Part model, mm, in its own coordinate system. A direction names the side the tool comes from. Round coordinates to 2 decimals unless told otherwise and drop trailing zeros. Loops run counter-clockwise (first coordinate to the right, second up) from the corner with the lowest first, then second, coordinate; pieces in that order, holes last. Notation, with made-up numbers: M -16.5,53.5 L 1.5,53.5 A20 ccw 1.5,74.5 Z; hole C 44.25,13.25 d1. An arc over 180 degrees is marked long. Put each result on its own line as item: value. Start each with the question number.
```python
from build123d import *
from build123d.topology import SkipClean

# Parameters (mm, degrees)
SKETCH_1_W          = 60
SKETCH_1_H          = 20
SKETCH_1_R          = 2.75
SKETCH_1_R_2        = 1.75
EXTRUDE_1_DEPTH     = 4
SKETCH_2_W          = 4
SKETCH_2_H          = 20
EXTRUDE_2_DEPTH     = 24
EXTRUDE_3_DEPTH     = 4
EXTRUDE_4_DEPTH     = 4
EXTRUDE_START       = 15
SKETCH_5_W          = 45
SKETCH_5_H          = 20
SKETCH_5_R          = 1.75
EXTRUDE_5_DEPTH     = 15
SKETCH_6_W          = 40
SKETCH_6_H          = 12
CUT_EXTRUDE_1_DEPTH = 15
SKETCH_7_R          = 2.75
CUT_EXTRUDE_2_DEPTH = 15
CUT_EXTRUDE_3_REACH = 76.303
SKETCH_8_W          = 30
SKETCH_8_H          = 20
SKETCH_10_W         = 26
SKETCH_10_H         = 12
EXTRUDE_6_DEPTH     = 4
SKETCH_11_W         = 15
SKETCH_11_H         = 12
EXTRUDE_7_DEPTH     = 4


with BuildPart() as part:
    # 草图1 → 凸台-拉伸1 (new body)
    with BuildSketch(Plane.XY):
        with Locations((30, -10)):
            Rectangle(SKETCH_1_W, SKETCH_1_H)
        with Locations((5, -5)):
            Circle(SKETCH_1_R, mode=Mode.SUBTRACT)
        with Locations((5, -15)):
            Circle(SKETCH_1_R, mode=Mode.SUBTRACT)
        with Locations((55, -10)):
            Circle(SKETCH_1_R_2, mode=Mode.SUBTRACT)
    extrude(amount=EXTRUDE_1_DEPTH)

    # 草图2 → 凸台-拉伸2 (add)
    with BuildSketch(Plane(origin=(0, 0, 0), x_dir=(-1, 0, 0), z_dir=(0, 0, -1))):
        with Locations((-17, -10)):
            Rectangle(SKETCH_2_W, SKETCH_2_H)
    extrude(amount=-EXTRUDE_2_DEPTH)

    # 草图3 → 凸台-拉伸3 (add)
    with BuildSketch(Plane.XZ.offset(20)):
        Polygon((19, 24), (60, 4), (19, 4), align=None)
    extrude(amount=-EXTRUDE_3_DEPTH)

    # 草图4 → 凸台-拉伸4 (add)
    with BuildSketch(Plane(origin=(0, 0, 0), x_dir=(1, 0, 0), z_dir=(0, 1, 0))):
        Polygon((19, -24), (60, -4), (19, -4), align=None)
    extrude(amount=-EXTRUDE_4_DEPTH)

    # 草图5 → 凸台-拉伸5 (add)
    with SkipClean():  # the faces are left unmerged after this step: merging them gives an invalid solid
        with BuildSketch(Plane(origin=(0, 0, 0), x_dir=(-1, 0, 0), z_dir=(0, 0, -1)).offset(EXTRUDE_START)):
            with Locations((-37.5, -10)):
                Rectangle(SKETCH_5_W, SKETCH_5_H)
            with Locations((-55, -10)):
                Circle(SKETCH_5_R, mode=Mode.SUBTRACT)
        extrude(amount=-EXTRUDE_5_DEPTH)

    # 草图6 → 切除-拉伸1 (cut)
    with BuildSketch(Plane.XY.offset(4)):
        with Locations((40, -10)):
            Rectangle(SKETCH_6_W, SKETCH_6_H)
    extrude(amount=-CUT_EXTRUDE_1_DEPTH, mode=Mode.SUBTRACT)

    # 草图7 → 切除-拉伸2 (cut)
    with BuildSketch(Plane(origin=(19, 0, 0), x_dir=(0, 0, -1), z_dir=(1, 0, 0))):
        with Locations(Location((-14, -10, 0), (0, 0, 90))):
            Circle(SKETCH_7_R)
    extrude(amount=-CUT_EXTRUDE_2_DEPTH, mode=Mode.SUBTRACT)

    # 切除-拉伸3: up to this face of the body (flat: up to its plane)
    cut_extrude_3_end = Plane(part.part.faces().sort_by_distance((7.970492187, -10, 0))[0])
    # 草图8 → 切除-拉伸3 (cut, up to the picked face)
    with BuildSketch(Plane(origin=(0, 0, -15), x_dir=(-1, 0, 0), z_dir=(0, 0, -1)), mode=Mode.PRIVATE) as cut_extrude_3_sk1:
        with Locations((-30, -10)):
            Rectangle(SKETCH_8_W, SKETCH_8_H)
    cut_extrude_3_tool1 = split(extrude(cut_extrude_3_sk1.sketch, amount=-CUT_EXTRUDE_3_REACH, mode=Mode.PRIVATE), bisect_by=cut_extrude_3_end, keep=Keep.BOTH, mode=Mode.PRIVATE)
    add(cut_extrude_3_tool1.solids().sort_by(Axis((30, -10, -15), (0, 0, 1)))[0], mode=Mode.SUBTRACT)

    # 草图10 → 凸台-拉伸6 (add)
    with BuildSketch(Plane.XY.offset(4)):
        with Locations((32, -10)):
            Rectangle(SKETCH_10_W, SKETCH_10_H)
    extrude(amount=-EXTRUDE_6_DEPTH)

    # 草图11 → 凸台-拉伸7 (add)
    with BuildSketch(Plane(origin=(45, 0, 0), x_dir=(0, 0, -1), z_dir=(1, 0, 0))):
        with Locations((3.5, -10)):
            Rectangle(SKETCH_11_W, SKETCH_11_H)
    extrude(amount=EXTRUDE_7_DEPTH)


solid = part.part
```
1. Cut at D-D, the plane x = 17. Give the cut face in (y, z), and give its area (3 significant figures).
2. Wall check: L1, parallel to Y at x = 5, z = 1.7; L2, parallel to Y at x = 33, z = 6.5; L3, parallel to Y at x = 55, z = -12.2. Give the ranges that are in metal, low to high.
3. Mould opens along X. For faces 1 (the cylindrical face through (17.028, -10.358, 16.727)), 2 (the cylindrical face through (7.62, -14.17, 1.97)), 3 (the flat face through (39.21, -18.03, 14.14)) say: released by +X, released by -X, zero draft, split by the parting line, or undercut.
4. Drop flat-ended pins along their axis: pin 1 (17.5 mm diameter, centred on x = 49, z = 15, fed in from -Y); pin 2 (7.5 mm diameter, centred on y = -6.5, z = -11, fed in from -X); pin 3 (8 mm diameter, centred on x = 32.5, y = -17, fed in from -Z); pin 4 (6 mm diameter, centred on y = -14, z = 11, fed in from -X). Give the stop position or say it passes through.
5. Cut at C-C, the plane y = -6.25. Give the cut face in (x, z), and give its area (3 significant figures).
6. Cut at B-B, the plane z = 14. Give the cut face in (x, y).
7. Which spindle directions (+Z, -Z, +X, -X, +Y, -Y) get a long thin tool onto all of the face, cutting with end or side? Do faces 4 (the flat face through (39, -16, 7)), 5 (the flat face through (22, -10, 0)), 6 (the flat face through (7, -10, 4)). Say none if no direction does.
8. Cut at A-A, the plane x = 5. Give the cut face in (y, z).
Results list:
1. outline: M -20,0 L 0,0 L 0,24 L -20,24 Z; hole C -10,14 d5.5
1. area: 456 mm^2
2. L1: y = -20 to -17.75, -12.25 to -7.75, -2.25 to 0
2. L2: y = -20 to -16, -4 to 0
2. L3: y = -20 to -11.75, -8.25 to 0
3. face 1: zero draft
3. face 2: undercut
3. face 3: released by +X
4. pin 1: stops at y = -20
4. pin 2: stops at x = 45
4. pin 3: stops at z = 0
4. pin 4: stops at x = 15
5. outline: M 0,0 L 2.55,0 L 2.55,4 L 0,4 Z; M 7.45,0 L 45,0 L 45,-15 L 60,-15 L 60,-11 L 49,-11 L 49,4 L 19,4 L 19,24 L 15,24 L 15,4 L 7.45,4 Z
5. area: 360 mm^2
6. outline: M 15,-20 L 39.5,-20 L 39.5,-16 L 19,-16 L 19,-12.75 L 15,-12.75 Z; M 15,-7.25 L 19,-7.25 L 19,-4 L 39.5,-4 L 39.5,0 L 15,0 Z
7. face 4: +Z, +X
7. face 5: -Z, -X, +Y, -Y
7. face 6: +Z, -X, +Y, -Y
8. outline: M -20,0 L -17.75,0 L -17.75,4 L -20,4 Z; M -12.25,0 L -7.75,0 L -7.75,4 L -12.25,4 Z; M -2.25,0 L 0,0 L 0,4 L -2.25,4 Z
